```python
from build123d import *

# Parameters (mm, degrees)
F2_DEPTH  = 60
F4_DEPTH  = 15
F6_DEPTH  = 60.001
F9_DEPTH  = 30.001
F10_R     = 5
F11_DEPTH = 15


with BuildPart() as f2:
    # F1 (on Front) → F2 (new body)
    with BuildSketch(Plane.XZ):
        with BuildLine():
            ThreePointArc((30, 0), (0, 30), (-30, 0))
            Line((-30, 0), (30, 0))
        make_face()
    extrude(amount=F2_DEPTH)

    # F3 (on Top) → F4 (join)
    with BuildSketch(Plane.XY):
        with BuildLine():
            Line((40, 0), (-40, 0))
            ThreePointArc((-40, 0), (-50, -10), (-40, -20))
            Line((-40, -20), (40, -20))
            ThreePointArc((40, -20), (50, -10), (40, 0))
        make_face()
    extrude(amount=F4_DEPTH)

    # F5 (on Front) → F6 (cut, through all)
    with BuildSketch(Plane.XZ):
        with BuildLine():
            ThreePointArc((25, 0), (0, 25), (-25, 0))
            Line((-25, 0), (25, 0))
        make_face()
    extrude(amount=F6_DEPTH, mode=Mode.SUBTRACT)

    # F8 (on offset) → F9 (cut, through all)
    with BuildSketch(Plane.XY.offset(30)):
        with BuildLine():
            Line((-10, -60), (0, -60))
            Line((0, -60), (10, -60))
            Line((10, -60), (10, -40))
            ThreePointArc((10, -40), (0, -30), (-10, -40))
            Line((-10, -40), (-10, -60))
        make_face()
    extrude(amount=-F9_DEPTH, mode=Mode.SUBTRACT)

    # F10 (on Top) → F11 (cut, through all)
    with BuildSketch(Plane.XY):
        with Locations((-40, -10.4273502391)):
            Circle(F10_R)
        with Locations((40, -10.0854694971)):
            Circle(F10_R)
    extrude(amount=F11_DEPTH, mode=Mode.SUBTRACT)


solid = f2.part
```
Geometry: final body of the model. Coordinates: model frame, mm. A direction names the side the tool comes from. Give positions to 0.01 mm unless a question says otherwise; leave off trailing zeros. Write each loop counter-clockwise with the first axis right and the second up, starting at its lowest first coordinate (ties: lowest second). Pieces come first, ordered by that corner, then holes.
1. Draft query along X for faces 1 (the flat face through (34, -20, 7)), 2 (the cylindrical face through (0, -30, 27)), 3 (the cylindrical face through (0.66, -29.58, 29.993)). Return one class per face: released by +X, released by -X, zero draft, split by the parting line, or undercut.
2. Section query D-D, the plane x = -33.5. Return loops of the section in (y, z).
3. Reachability of faces 4 (the flat face through (35, -8, 15)), 5 (the cylindrical face through (0.55, -29.58, 24.994)), 6 (the flat face through (10, -50, 26)), 7 (the flat face through (-35, -20, 7)), 8 (the flat face through (-35, -8, 15)) from +Z, -Z, +X, -X, +Y, -Y: full face, straight path, thin tool, end or side. Return the list, or none.
4. Pin query (flat end, axial travel): P1, Ø7, axis at x = 33.5, z = 9.5, coming from the -Y side; P2, Ø2, axis at y = -21.5, z = 23.5, coming from the +X side; P3, Ø9, axis at x = -40, y = -10.43, coming from the -Z side; P4, Ø13, axis at x = 40, y = -10.09, coming from the +Z side. Return the tip coordinate at first contact, or that it passes through.
5. Section query B-B, the plane z = 12. Return loops of the section in (x, y).
6. Section query A-A, the plane y = -31. Return loops of the section in (x, z), then the cut area to 3 significant figures.
7. Line query: probe 1 along Y at (x, z) = (40, 5); probe 2 along X at (y, z) = (-30.5, 14); probe 3 along X at (y, z) = (-54, 21). Output: solid intervals per line, ascending.
8. Section query C-C, the plane z = 19. Return loops of the section in (x, y), then the cut area to 3 significant figures.
Computed:
1. face 1: zero draft
1. face 2: undercut
1. face 3: split by the parting line
2. outline: (-20, 0) - (0, 0) - (0, 15) - (-20, 15) - close
3. face 4: +Z, +X, +Y, -Y
3. face 5: -Z, +Y, -Y
3. face 6: +Z, -Z, -Y
3. face 7: +Z, -X, -Y
3. face 8: +Z, -X, +Y, -Y
4. P1: stops at y = -20
4. P2: stops at x = 19.84
4. P3: passes through
4. P4: stops at z = 15
5. outline: (-40, -20) - (-27.5, -20) - (-27.5, -60) - (-21.93, -60) - (-21.93, 0) - (-40, 0) arc R10 ccw to start; (21.93, -60) - (27.5, -60) - (27.5, -20) - (40, -20) arc R10 ccw to (40, 0) - (21.93, 0) - close; hole circle Ø10 at (-40, -10.43); hole circle Ø10 at (40, -10.09)
6. outline: (-30, 0) - (-25, 0) arc R25 cw to (-4.36, 24.62) - (-4.36, 29.68) arc R30 ccw to start; (4.36, 24.62) arc R25 cw to (25, 0) - (30, 0) arc R30 ccw to (4.36, 29.68) - close
6. area: 388 mm2
7. probe 1: y = -20 to -15.09, -5.09 to 0
7. probe 2: x = -26.53 to -20.71, 20.71 to 26.53
7. probe 3: x = -21.42 to -13.56, 13.56 to 21.42
8. outline: (-23.22, -60) - (-16.25, -60) - (-16.25, 0) - (-23.22, 0) - close; (16.25, -60) - (23.22, -60) - (23.22, 0) - (16.25, 0) - close
8. area: 836 mm2
